Build history of the part. All positions in model axes, mm. Face numbers are marked on the shaded views. A direction names the side the tool comes from. Coordinates: 2 decimals unless noted, no trailing zeros. Loops run counter-clockwise (first coordinate to the right, second up) from the corner with the lowest first, then second, coordinate; pieces in that order, holes last.
(1) Two-plate mould, pull along Y, no slides. Class the marked faces 1, 2 and 3: pulls with the +Y half, pulls with the -Y half, needs draft (parallel to the pull), parting line crosses it, or undercut.
(2) Slice it at A-A (y = -3.5). Give the cut face in (x, z), and give its area (3 significant figures).
(3) Wall check: L1, parallel to X at y = -3.55, z = 0; L2, parallel to Y at x = 4.25, z = -2.75; L3, parallel to X at y = 4.5, z = 0. Give the ranges that are in metal, low to high.
(4) Tool access for the marked faces 4, 5 and 6: list every direction of +Z, -Z, +X, -X, +Y, -Y with a clear straight run to the whole face (end or side of a thin tool).
(5) Flat gauge pins, fed straight in: P1, Ø4, axis at x = 0, z = 0, coming from the +Y side; P2, Ø6.5, axis at x = 0, z = 0, coming from the -Y side. Where does each tip first touch, or does it go through?
from build123d import *

# Parameters (mm, degrees)
ESTRUSIONE_ESTRUSIONE1_OUTLINE_R = 2.5
ESTRUSIONE_ESTRUSIONE1_DEPTH     = 6
SCHIZZO2_R                       = 7
ESTRUSIONE_ESTRUSIONE2_DEPTH     = 1
FORI_FILETTATI_5_0MM1_D          = 5
ESTRUSIONE_ESTRUSIONE3_START     = 6
SCHIZZO4_R                       = 7
ESTRUSIONE_ESTRUSIONE3_DEPTH     = 6
FORI_FILETTATI_5_0MM2_D          = 5
FORI_FILETTATI_5_0MM2_DEPTH      = 10
FORI_FILETTATI_5_0MM2_TIP        = 1.502151548


# Read off the part's stored shape, not the designer's step: Estrusione-Estrusione1
with BuildPart() as part:
    # Estrusione-Estrusione1 outline → Estrusione-Estrusione1 (new body)
    with BuildSketch(Plane(origin=(0, 0, 0), x_dir=(1, 0, 0), z_dir=(0, 1, 0))):
        Polygon((-4.558413324, 4.655107649), (-5.141001385, 4.002407278), (-4.021493725, 3.00315582), (-4.481890734, 2.259206078), (-5.875647949, 2.815301129), (-6.199864976, 2.002706553), (-4.806107761, 1.446611503), (-4.984293637, 0.590062369), (-6.484192715, 0.635927742), (-6.51093335, -0.238550138), (-5.011034272, -0.284415511), (-4.885517166, -1.15025157), (-6.310648144, -1.620147915), (-6.036687071, -2.451034162), (-4.611556094, -1.981137817), (-4.197475223, -2.751828193), (-5.375946271, -3.680809823), (-4.83432724, -4.367887293), (-3.655856192, -3.438905663), (-3.00315582, -4.021493725), (-3.792825937, -5.297511743), (-3.048876196, -5.757908753), (-2.259206078, -4.481890734), (-1.446611503, -4.806107761), (-1.75223482, -6.275255564), (-0.895685686, -6.45344144), (-0.590062369, -4.984293637), (0.284415511, -5.011034272), (0.499701678, -6.496110952), (1.365537736, -6.370593846), (1.15025157, -4.885517166), (1.981137817, -4.611556094), (2.691366778, -5.933439486), (3.462057155, -5.519358615), (2.751828193, -4.197475223), (3.438905663, -3.655856192), (4.558413324, -4.655107649), (5.141001385, -4.002407278), (4.021493725, -3.00315582), (4.481890734, -2.259206078), (5.875647949, -2.815301129), (6.199864976, -2.002706553), (4.806107761, -1.446611503), (4.984293637, -0.590062369), (6.484192715, -0.635927742), (6.51093335, 0.238550138), (5.011034272, 0.284415511), (4.885517166, 1.15025157), (6.310648144, 1.620147915), (6.036687071, 2.451034162), (4.611556094, 1.981137817), (4.197475223, 2.751828193), (5.375946271, 3.680809823), (4.83432724, 4.367887293), (3.655856192, 3.438905663), (3.00315582, 4.021493725), (3.792825937, 5.297511743), (3.048876196, 5.757908753), (2.259206078, 4.481890734), (1.446611503, 4.806107761), (1.75223482, 6.275255564), (0.895685686, 6.45344144), (0.590062369, 4.984293637), (-0.284415511, 5.011034272), (-0.499701678, 6.496110952), (-1.365537736, 6.370593846), (-1.15025157, 4.885517166), (-1.981137817, 4.611556094), (-2.691366778, 5.933439486), (-3.462057155, 5.519358615), (-2.751828193, 4.197475223), (-3.438905663, 3.655856192), align=None)
        Circle(ESTRUSIONE_ESTRUSIONE1_OUTLINE_R, mode=Mode.SUBTRACT)
    extrude(amount=ESTRUSIONE_ESTRUSIONE1_DEPTH)

    # Schizzo2 → Estrusione-Estrusione2 (add)
    with BuildSketch(Plane(origin=(0, 6, 0), x_dir=(1, 0, 0), z_dir=(0, 1, 0))):
        with Locations(Location((0, 0, 0), (0, 0, 270))):
            Circle(SCHIZZO2_R)
    extrude(amount=ESTRUSIONE_ESTRUSIONE2_DEPTH)

    # Fori filettati Ø5.0mm1 (through all)
    with Locations(Plane.ZX.offset(7)):
        with Locations((0, 0)):
            Hole(FORI_FILETTATI_5_0MM1_D / 2)

    # Schizzo4 → Estrusione-Estrusione3 (add)
    with BuildSketch(Plane.XZ.offset(ESTRUSIONE_ESTRUSIONE3_START)):
        with Locations(Location((0, 0, 0), (0, 0, 90))):
            Circle(SCHIZZO4_R)
    extrude(amount=-ESTRUSIONE_ESTRUSIONE3_DEPTH)

    # Fori filettati Ø5.0mm2
    with Locations(Plane(origin=(0, -6, 0), x_dir=(0, 0, -1), z_dir=(0, -1, 0))):
        with Locations((0, 0)):
            Hole(FORI_FILETTATI_5_0MM2_D / 2, depth=FORI_FILETTATI_5_0MM2_DEPTH)
            with Locations((0, 0, -(FORI_FILETTATI_5_0MM2_DEPTH + FORI_FILETTATI_5_0MM2_TIP / 2))):  # 118° drill point
                Cone(0, FORI_FILETTATI_5_0MM2_D / 2, FORI_FILETTATI_5_0MM2_TIP, mode=Mode.SUBTRACT)


solid = part.part
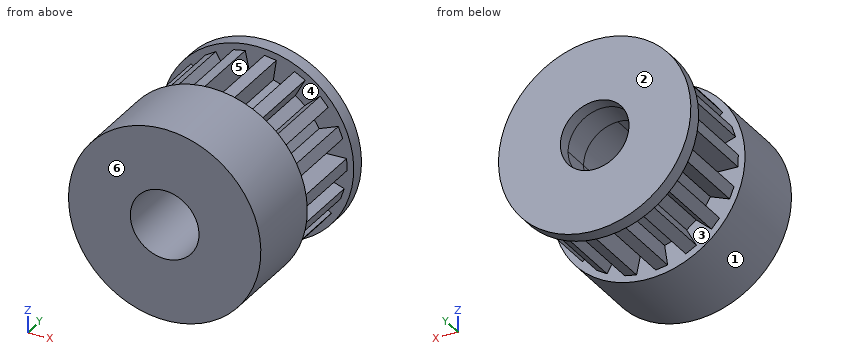
Response values:
1. face 1: needs draft
1. face 2: pulls with the +Y half
1. face 3: undercut
2. outline: circle Ø14 at (0, 0); hole circle Ø5 at (0, 0)
2. area: 134 mm2
3. L1: x = -7 to -2.5, 2.5 to 7
3. L2: y = -6 to 0, 6 to 7
3. L3: x = -6.5 to -2.5, 2.5 to 6.5
4. face 4: none
4. face 5: +Z
4. face 6: +Z, -Z, +X, -X, -Y
5. P1: passes through
5. P2: stops at y = -6
